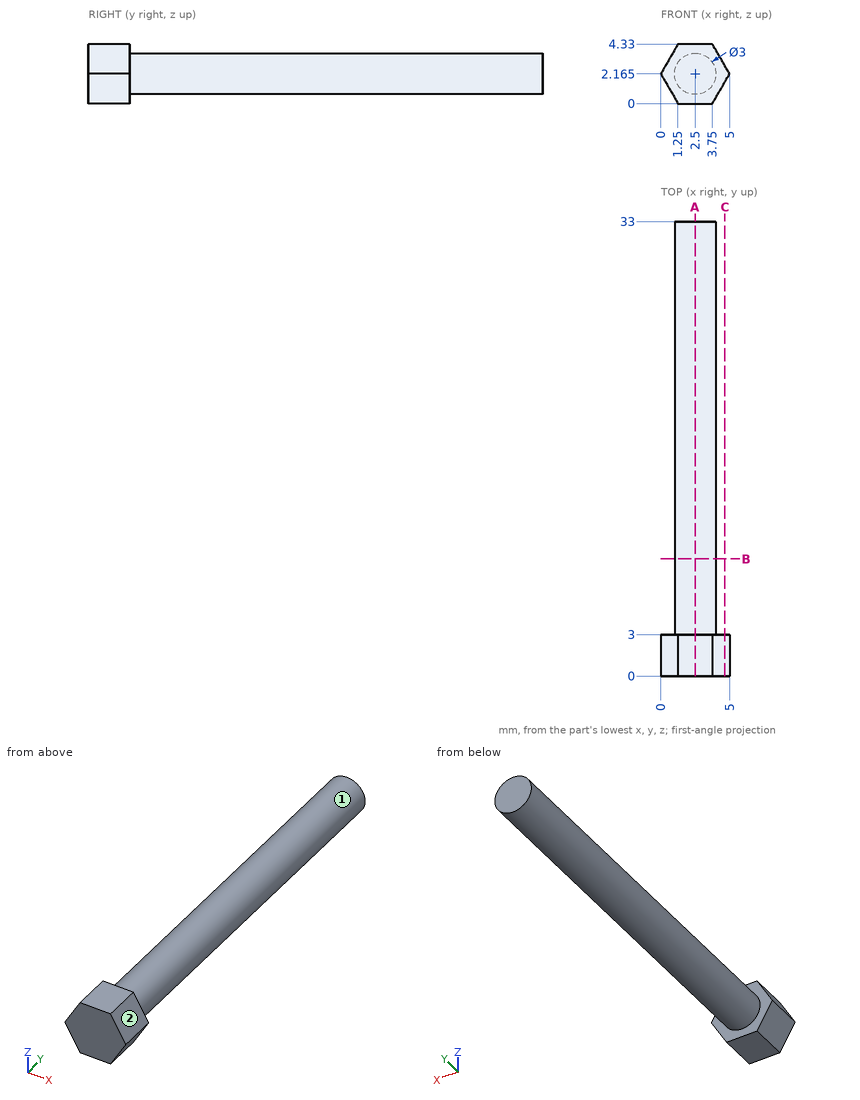
Check sheet for the drawn part. Datum: minimum x, y, z corner. Units: mm. A direction names the side the tool comes from. Give positions to 0.01 mm unless a question says otherwise; leave off trailing zeros. Write each loop counter-clockwise with the first axis right and the second up, starting at its lowest first coordinate (ties: lowest second). Pieces come first, ordered by that corner, then holes. Notation, with made-up numbers: (-37.75, -39) -> (4.25, -39) arc R29 cw to (4.25, -16) -> close; hole circle Ø7 at (0.25, -35.5). An arc over 180 degrees is marked (long way). Use one line per item in the form item = value. Start each with the question number.
1. Thickness scan on line 1 along Y through (x, z) = (0.7, 1.6); line 2 along Z through (x, y) = (2.35, 6.5); line 3 along X through (y, z) = (4, 2.15). Record the ranges inside material, lowest first. Write a range as from..to.
2. Go/stop test with flat-tipped pins: P1, Ø2, axis at x = 3.5, y = 22.5, coming from the -Z side (3 decimals); P2, Ø1, axis at x = 4, y = 26, coming from the -Z side. Record where each tip stops, or that it passes through.
3. Access from +Z, -Z, +X, -X, +Y, -Y to the whole of each face (thin tool, end or side, straight path). Record for the marked faces 1 and 2.
4. Section check C-C (x = 4.65). Record the cut outline in (y, z).
5. Section check B-B (y = 8.5). Record the cut outline in (x, z) (3 decimals), and give its area (3 significant figures).
6. Section check A-A (x = 2.5). Record the cut outline in (y, z) (3 decimals).
Conclusion:
q1.line_1 = 0..3
q1.line_2 = 0.67..3.66
q1.line_3 = 1..4
q2.P1 = 0.665
q2.P2 = 1.05
q3.face_1 = +Y
q3.face_2 = +Z, +X, +Y, -Y
q4.outline = (0, 1.56) -> (3, 1.56) -> (3, 2.77) -> (0, 2.77) -> close
q5.outline = circle Ø3 at (2.5, 2.165)
q5.area = 7.07 mm²
q6.outline = (0, 0) -> (3, 0) -> (3, 0.665) -> (33, 0.665) -> (33, 3.665) -> (3, 3.665) -> (3, 4.33) -> (0, 4.33) -> close
